The model under review builds one solid part; all positions refer to its coordinate system, in mm. A direction names the side the tool comes from. Give positions to 0.01 mm unless a question says otherwise; leave off trailing zeros. Order: outer loops, then holes, each group sorted by start corner. A loop starts at its lowest first (then second) coordinate and runs counter-clockwise, first axis right, second up. Notation, with made-up numbers: (24, 33) - (43, 33) arc R13 cw to (43, 55) - close; hole circle Ø9 at (89.5, 52). An arc over 180 degrees is marked (long way). Use CSV: the item, a comma, the result in double quotes. Start each with the question number.
```python
from build123d import *

# Parameters (mm, degrees)
F0_R     = 1.5
F1_DEPTH = 3
F3_START = 18.5
F2_W     = 16.5
F2_H     = 17
F2_R     = 3.3
F3_DEPTH = 3.5
F4_R     = 2


with BuildPart() as f1:
    # F0 (on Top) → F1 (new body)
    with BuildSketch(Plane.XY):
        with BuildLine():
            Line((26.25, 0), (1, 0))
            ThreePointArc((1, 0), (0.2928932188, -0.2928932188), (0, -1))
            Line((0, -1), (0, -40.9))
            Line((0, -40.9), (26.25, -40.9))
            Line((26.25, -40.9), (26.25, 0))
        make_face()
        with Locations((4.5, -4.5)):
            Circle(F0_R, mode=Mode.SUBTRACT)
        with BuildLine():
            Line((51.5, 0), (26.25, 0))
            Line((26.25, 0), (26.25, -40.9))
            Line((26.25, -40.9), (52.5, -40.9))
            Line((52.5, -40.9), (52.5, -1))
            ThreePointArc((52.5, -1), (52.2071067812, -0.2928932188), (51.5, 0))
        make_face()
        with Locations((48, -4.5)):
            Circle(F0_R, mode=Mode.SUBTRACT)
        with BuildLine():
            Line((52.5, -40.9), (26.25, -40.9))
            Line((26.25, -40.9), (26.25, -81.8))
            Line((26.25, -81.8), (33.997034058, -81.8))
            Line((33.997034058, -81.8), (51.5, -81.8))
            ThreePointArc((51.5, -81.8), (52.2071067812, -81.5071067812), (52.5, -80.8))
            Line((52.5, -80.8), (52.5, -40.9))
        make_face()
        with BuildLine():
            Line((26.25, -81.8), (26.25, -40.9))
            Line((26.25, -40.9), (0, -40.9))
            Line((0, -40.9), (0, -80.8))
            ThreePointArc((0, -80.8), (0.2928932188, -81.5071067812), (1, -81.8))
            Line((1, -81.8), (18.997034058, -81.8))
            Line((18.997034058, -81.8), (26.25, -81.8))
        make_face()
        with BuildLine():
            Line((26.25, -85.8), (26.25, -81.8))
            Line((26.25, -81.8), (18.997034058, -81.8))
            Line((18.997034058, -81.8), (18.997034058, -84.8))
            ThreePointArc((18.997034058, -84.8), (19.2899272768, -85.5071067812), (19.997034058, -85.8))
            Line((19.997034058, -85.8), (26.25, -85.8))
        make_face()
        with BuildLine():
            Line((33.997034058, -81.8), (26.25, -81.8))
            Line((26.25, -81.8), (26.25, -85.8))
            Line((26.25, -85.8), (32.997034058, -85.8))
            ThreePointArc((32.997034058, -85.8), (33.7041408392, -85.5071067812), (33.997034058, -84.8))
            Line((33.997034058, -84.8), (33.997034058, -81.8))
        make_face()
    extrude(amount=-F1_DEPTH)

    # F2 (on Right) → F3 (join)
    with BuildSketch(Plane.YZ.offset(F3_START)):
        with Locations((-40.9, 8.5)):
            Rectangle(F2_W, F2_H)
        with Locations((-40.9, 8.5)):
            Circle(F2_R, mode=Mode.SUBTRACT)
    extrude(amount=F3_DEPTH)

    # F4
    f4_edges = [f1.edges().sort_by_distance(p)[0] for p in [
        (20.25, -49.15, 17),
        (20.25, -32.65, 17),
    ]]
    fillet(f4_edges, radius=F4_R)


solid = f1.part
```
1. Consider section A-A (z = 8.5). Give the boundary of the cut face in (x, y).
2. Mouldability with a two-part tool opening along Y and no side actions: class faces 1 (the face through (26, -85.8, -1)), 2 (the face through (5.93, -4.05, -1.48)), 3 (the face through (20, -41, 17)) as pulls with the +Y half, pulls with the -Y half, needs draft (parallel to the pull), parting line crosses it, or undercut.
3. To check wall thickness, follow L1, parallel to Y at x = 4.5, z = -1.6; L2, parallel to Z at x = 42, y = -11; L3, parallel to X at y = -48, z = 9.75. State the ranges of each line that lie inside material, in increasing order. Write a range as [from, to].
4. Consider section C-C (x = 48). Give the boundary of the cut face in (y, z).
5. Clearance check with flat-ended pins moving along their axes: pin 1 (1 mm diameter, centred on x = 16.5, y = -41, fed in from +Z); pin 2 (2.5 mm diameter, centred on y = -83.5, z = -1, fed in from -X); pin 3 (1.5 mm diameter, centred on x = 13.5, z = -1.5, fed in from -Y); pin 4 (5.5 mm diameter, centred on y = -40.9, z = 8.5, fed in from -X). State where each tip first meets the part, or that it passes through.
6. Tool access review of faces 4 (the face through (43, -81.8, -1)), 5 (the face through (18.5, -37, 9)), 6 (the face through (22, -37, 9)), 7 (the face through (20, -32.65, 7)): name each direction out of +Z, -Z, +X, -X, +Y, -Y from which nothing blocks a thin tool from reaching the whole face with its end or side.
7. Consider section B-B (y = -4.5). Give the boundary of the cut face in (x, z), and give its area (4 significant figures).
8. Consider section D-D (x = 15). Give the boundary of the cut face in (y, z).
Answers follow:
1,outline,"(18.5, -49.15) - (22, -49.15) - (22, -44.2) - (18.5, -44.2) - close; (18.5, -37.6) - (22, -37.6) - (22, -32.65) - (18.5, -32.65) - close"
2,face 1,"pulls with the -Y half"
2,face 2,"undercut"
2,face 3,"needs draft"
3,L1,"y = [-81.8, -6], [-3, 0]"
3,L2,"z = [-3, 0]"
3,L3,"x = [18.5, 22]"
4,outline,"(-81.8, -3) - (-6, -3) - (-6, 0) - (-81.8, 0) - close; (-3, -3) - (0, -3) - (0, 0) - (-3, 0) - close"
5,pin 1,"stops at z = 0"
5,pin 2,"stops at x = 19"
5,pin 3,"stops at y = -81.8"
5,pin 4,"passes through"
6,face 4,"+Z, -Z, +X, -Y"
6,face 5,"+Z, -X, +Y, -Y"
6,face 6,"+Z, +X, +Y, -Y"
6,face 7,"+Z, +X, -X, +Y"
7,outline,"(0, -3) - (3, -3) - (3, 0) - (0, 0) - close; (6, -3) - (46.5, -3) - (46.5, 0) - (6, 0) - close; (49.5, -3) - (52.5, -3) - (52.5, 0) - (49.5, 0) - close"
7,area,"139.5 mm^2"
8,outline,"(-81.8, -3) - (0, -3) - (0, 0) - (-81.8, 0) - close"
